Autodesk Fusion 360 part; units mm, degrees
sketch "Sketch1" plane through (0, 0, 0) normal (0, 0, 1) x (1, 0, 0)
  circle A0 centre (0, 0) radius 4
  circle A1 centre (0, 0) radius 6
  dimension "d1" = 8
  dimension "d2" = 12
extrude "Extrude1" add sketch "Sketch1" along normal blind 5 makes body 1
copy_body "Body->Comp1" bodies 1 removing the originals makes body 2 in component "5mm Spacer - 8mm Shaft"
component "5mm Spacer - 8mm Shaft" placed x (1, 0, 0) y (0, 1, 0) z (0, 0, 1) at (0, 0, 0)
For this review, take the finished solid that the model builds, in its own axes (mm). Round coordinates to 2 decimals unless told otherwise and drop trailing zeros. Loops run counter-clockwise (first coordinate to the right, second up) from the corner with the lowest first, then second, coordinate; pieces in that order, holes last. Notation, with made-up numbers: (-37.5, 42.25) - (-24.5, 42.25) arc R11 ccw to (-24.5, 51.25) - close; hole circle Ø9 at (18.5, 35). An arc over 180 degrees is marked (long way). Put each result on its own line as item: value. Start each with the question number.
1. Mouldability with a two-part tool opening along X and no side actions: class faces 1 (the cylindrical face through (-0.867, 3.905, 2.465)), 2 (the flat face through (-1.42, -3.92, 0)), 3 (the cylindrical face through (-6, 0, 2)) as +X half, -X half, draft (parallel to the pull), parting line (faces both ways), or undercut.
2. Consider section A-A on y = 0. State the section outline as (x, z) points.
3. For probe 1 along Y at (x, z) = (0, 3.25); probe 2 along X at (y, z) = (3.25, 2.8); probe 3 along Y at (x, z) = (-1.75, 3.7), list the stretches that pass through material, from the lowest coordinate up. Write a range as [from, to].
4. Consider section C-C on z = 1.6. State the section outline as (x, y) points, plus the area to 3 significant figures.
5. Insertion check: P1, Ø2, axis at y = 2, z = 2, coming from the -X side; P2, Ø1.5, axis at y = 4, z = 4, coming from the +X side; P3, Ø1.5, axis at x = -2, z = 1, coming from the +Y side. Each pin has a flat end and moves straight along its axis. Give the tip position at first contact, or say it passes through.
Result sheet:
1. face 1: undercut
1. face 2: draft
1. face 3: parting line
2. outline: (-6, 0) - (-4, 0) - (-4, 5) - (-6, 5) - close; (4, 0) - (6, 0) - (6, 5) - (4, 5) - close
3. probe 1: [-6, -4], [4, 6]
3. probe 2: [-5.04, -2.33], [2.33, 5.04]
3. probe 3: [-5.74, -3.6], [3.6, 5.74]
4. outline: circle Ø12 at (0, 0); hole circle Ø8 at (0, 0)
4. area: 62.8 mm^2
5. P1: x = -5.92
5. P2: x = 5.04
5. P3: y = 5.87
